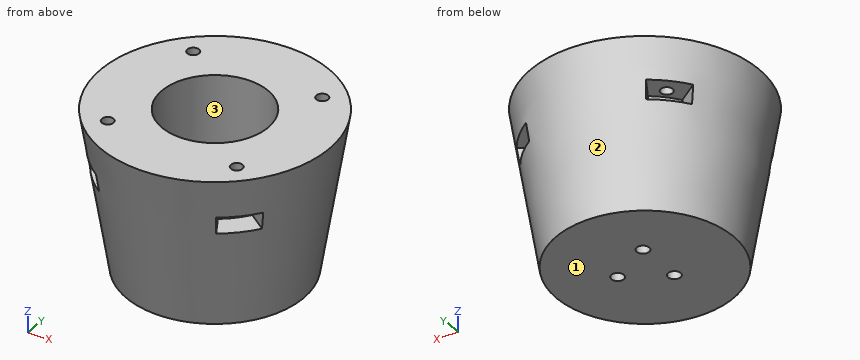
```python
from build123d import *

# Parameters (mm, degrees)
SKETCH1_R           = 29
BOSS_EXTRUDE1_DEPTH = 40
BOSS_EXTRUDE1_DRAFT = -9.23
SKETCH2_R           = 1.5
CUT_EXTRUDE1_DEPTH  = 10
SKETCH4_R           = 13.5
CUT_EXTRUDE3_DEPTH  = 35
SKETCH5_R           = 1.6
CUT_EXTRUDE4_DEPTH  = 35
CUT_EXTRUDE5_DEPTH  = 4.5


with BuildPart() as part:
    # Sketch1 → Boss-Extrude1 (with draft: the straight prism first)
    with BuildSketch(Plane.XY):
        Circle(SKETCH1_R)
    extrude(amount=-BOSS_EXTRUDE1_DEPTH)
    # Boss-Extrude1: the draft: its side faces are tilted about the plane it starts from
    boss_extrude1_sides = [part.faces().sort_by_distance(p)[0] for p in [
        (-29, 0, -20),
    ]]
    draft(boss_extrude1_sides, Plane.XY, BOSS_EXTRUDE1_DRAFT)

    # Sketch2 → Cut-Extrude1 (cut)
    with BuildSketch(Plane.XY):
        with Locations((-16.5, 16.5)):
            Circle(SKETCH2_R)
        with Locations(Location((16.5, 16.5, 0), (0, 0, 180))):
            Circle(SKETCH2_R)
        with Locations((16.5, -16.5)):
            Circle(SKETCH2_R)
        with Locations(Location((-16.5, -16.5, 0), (0, 0, 180))):
            Circle(SKETCH2_R)
    extrude(amount=-CUT_EXTRUDE1_DEPTH, mode=Mode.SUBTRACT)

    # Sketch4 → Cut-Extrude3 (cut)
    with BuildSketch(Plane.XY):
        Circle(SKETCH4_R)
    extrude(amount=-CUT_EXTRUDE3_DEPTH, mode=Mode.SUBTRACT)

    # Sketch5 → Cut-Extrude4 (cut)
    with BuildSketch(Plane.XY.offset(-35)):
        with Locations((7, 0)):
            Circle(SKETCH5_R)
        with Locations((-3.5, -6.062177826)):
            Circle(SKETCH5_R)
        with Locations((-3.5, 6.062177826)):
            Circle(SKETCH5_R)
    extrude(amount=-CUT_EXTRUDE4_DEPTH, mode=Mode.SUBTRACT)

    # Sketch6 → Cut-Extrude5 (cut)
    with BuildSketch(Plane.XY.offset(-10)):
        with BuildLine():
            Line((11.668923699, 17.275154255), (17.761390964, 25.810687075))
            ThreePointArc((17.761390964, 25.810687075), (22.367192771, 21.940083496), (26.14828814, 17.260521534))
            Line((26.14828814, 17.260521534), (17.027183551, 12.027874092))
            ThreePointArc((17.027183551, 12.027874092), (14.585956606, 14.894448789), (11.668923699, 17.275154255))
        make_face()
        with BuildLine():
            Line((12.027874092, -17.027183551), (17.260521534, -26.14828814))
            ThreePointArc((17.260521534, -26.14828814), (21.940083496, -22.367192771), (25.810687075, -17.761390964))
            Line((25.810687075, -17.761390964), (17.275154255, -11.668923699))
            ThreePointArc((17.275154255, -11.668923699), (14.894448789, -14.585956606), (12.027874092, -17.027183551))
        make_face()
        with BuildLine():
            Line((-17.027183551, -12.027874092), (-26.14828814, -17.260521534))
            ThreePointArc((-26.14828814, -17.260521534), (-22.367192771, -21.940083496), (-17.761390964, -25.810687075))
            Line((-17.761390964, -25.810687075), (-11.668923699, -17.275154255))
            ThreePointArc((-11.668923699, -17.275154255), (-14.585956606, -14.894448789), (-17.027183551, -12.027874092))
        make_face()
        with BuildLine():
            Line((-12.027874092, 17.027183551), (-17.260521534, 26.14828814))
            ThreePointArc((-17.260521534, 26.14828814), (-21.940083496, 22.367192771), (-25.810687075, 17.761390964))
            Line((-25.810687075, 17.761390964), (-17.275154255, 11.668923699))
            ThreePointArc((-17.275154255, 11.668923699), (-14.894448789, 14.585956606), (-12.027874092, 17.027183551))
        make_face()
    extrude(amount=-CUT_EXTRUDE5_DEPTH, mode=Mode.SUBTRACT)


solid = part.part
```
Verification items for the finished model (mm, model axes). Face numbers are marked on the shaded views. Round coordinates to 2 decimals unless told otherwise and drop trailing zeros. Order: outer loops, then holes, each group sorted by start corner. A loop starts at its lowest first (then second) coordinate and runs counter-clockwise, first axis right, second up. Notation, with made-up numbers: (37, 19) -> (53, 19) arc R10 ccw to (53, 38) -> close; hole circle Ø7 at (15, 2). An arc over 180 degrees is marked (long way). Put each result on its own line as item: value. Start each with the question number.
(1) Section check D-D (z = -23). Enter the section's corners in (x, y).
(2) Draft check along X on the marked faces 1, 2 and 3. Enter one of: +X half, -X half, draft (parallel to the pull), parting line (faces both ways), or undercut.
(3) Material ranges on line 1 along Y through (x, z) = (-16.5, -5.25); line 2 along Y through (x, z) = (-3, -37); line 3 along X through (y, z) = (16, -5), recorded low to high.
(4) Depth check by flat-ended pin: pin 1 Ø10 at (x, z) = (22, -36) entering from -Y; pin 2 Ø2.5 at (x, y) = (16.5, -16.5) entering from +Z; pin 3 Ø3.5 at (x, y) = (-3.5, 6.06) entering from +Z. Enter the tip coordinate at first touch or a pass-through.
(5) Section check B-B (z = -29). Enter the section's corners in (x, y), then the cut area to 3 significant figures.
(6) Section check A-A (z = -7.5). Enter the section's corners in (x, y), then the cut area to 3 significant figures.
(7) Section check C-C (x = -3.5). State how many separate pieces and enclosed holes the cut face has, then the cut area to 3 significant figures.
Completed:
1. outline: circle Ø50.52 at (0, 0); hole circle Ø27 at (0, 0)
2. face 1: draft
2. face 2: parting line
2. face 3: undercut
3. line 1: y = -22.8 to -18, -15 to 15, 18 to 22.8
3. line 2: y = -22.79 to -7.58, -4.54 to 4.54, 7.58 to 22.79
3. line 3: x = -23.21 to -17.91, -15.09 to 15.09, 17.91 to 23.21
4. pin 1: stops at y = -15.84
4. pin 2: stops at z = -14.5
4. pin 3: stops at z = -35
5. outline: circle Ø48.57 at (0, 0); hole circle Ø27 at (0, 0)
5. area: 1,280 mm2
6. outline: circle Ø55.56 at (0, 0); hole circle Ø3 at (-16.5, -16.5); hole circle Ø3 at (-16.5, 16.5); hole circle Ø27 at (0, 0); hole circle Ø3 at (16.5, -16.5); hole circle Ø3 at (16.5, 16.5)
6. area: 1,820 mm2
7. separate pieces: 3
7. enclosed holes: 0
7. area: 1,100 mm2
